from build123d import *

# Parameters (mm, degrees)
SKETCH2_R           = 22.5
SKETCH2_R_2         = 1.25
BOSS_EXTRUDE1_DEPTH = 10
SKETCH3_R           = 10
CUT_EXTRUDE1_DEPTH  = 4
FILLET1_R           = 2


with BuildPart() as part:
    # Sketch2 → Boss-Extrude1 (new body)
    with BuildSketch(Plane.XY):
        Circle(SKETCH2_R)
        with Locations((4, 0)):
            Circle(SKETCH2_R_2, mode=Mode.SUBTRACT)
        with Locations((0, 4)):
            Circle(SKETCH2_R_2, mode=Mode.SUBTRACT)
        with Locations((-4, 0)):
            Circle(SKETCH2_R_2, mode=Mode.SUBTRACT)
        with Locations((0, -4)):
            Circle(SKETCH2_R_2, mode=Mode.SUBTRACT)
    extrude(amount=BOSS_EXTRUDE1_DEPTH)

    # Sketch3 → Cut-Extrude1 (cut)
    with BuildSketch(Plane(origin=(0, 0, 0), x_dir=(-1, 0, 0), z_dir=(0, 0, -1))):
        Circle(SKETCH3_R)
    extrude(amount=-CUT_EXTRUDE1_DEPTH, mode=Mode.SUBTRACT)

    # Fillet1
    fillet1_edges = [part.edges().sort_by_distance(p)[0] for p in [
        (-22.5, 0, 0),
        (-22.5, 0, 10),
    ]]
    fillet(fillet1_edges, radius=FILLET1_R)


solid = part.part
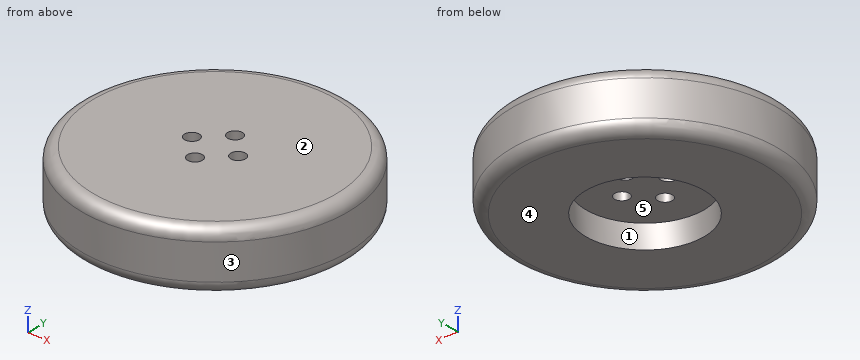
Build history of the part. All positions in model axes, mm. Face numbers are marked on the shaded views. A direction names the side the tool comes from. Round coordinates to 2 decimals unless told otherwise and drop trailing zeros. Write each loop counter-clockwise with the first axis right and the second up, starting at its lowest first coordinate (ties: lowest second). Pieces come first, ordered by that corner, then holes. Notation, with made-up numbers: M 40.5,0.5 L 90.5,0.5 A8 ccw 90.5,4.5 Z; hole C 21,-6.75 d8. An arc over 180 degrees is marked long. Answer as a JSON object with one key per item and string values. Group by question number.
(1) Which spindle directions (+Z, -Z, +X, -X, +Y, -Y) get a long thin tool onto all of the face, cutting with end or side? Do the marked faces 1 and 2. Say none if no direction does.
(2) Flat gauge pins, fed straight in: pin 1 (5 mm diameter, centred on x = 5.5, z = 2.5, fed in from -Y); pin 2 (1.5 mm diameter, centred on x = 0, y = 4, fed in from +Z); pin 3 (4 mm diameter, centred on x = -4, y = 0, fed in from -Z); pin 4 (6 mm diameter, centred on x = -16.5, z = 2, fed in from -Y). Where does each tip first touch, or does it go through?
(3) Mould opens along X. For the marked faces 3, 4 and 5 say: pulls with the +X half, pulls with the -X half, needs draft (parallel to the pull), parting line crosses it, or undercut.
(4) Cut at A-A (x = 0). Give the cut face in (y, z), and give its area (3 significant figures).
(5) Cut at C-C (z = 6.5). Give the cut face in (x, y).
(6) Drill centre lines: L1, parallel to Y at x = 0, z = 1.95; L2, parallel to Y at x = 0.5, z = 6; L3, parallel to Z at x = 9, y = -2. Where is each one in solid material? Low to high.
Responses:
{
 "1": {"face 1": "-Z", "face 2": "+Z, +X, -X, +Y, -Y"},
 "2": {"pin 1": "stops at y = -22.3", "pin 2": "passes through", "pin 3": "stops at z = 4", "pin 4": "stops at y = -18"},
 "3": {"face 3": "parting line crosses it", "face 4": "needs draft", "face 5": "undercut"},
 "4": {"outline": "M -22.5,2 A2 ccw -20.5,0 L -10,0 L -10,4 L -5.25,4 L -5.25,10 L -20.5,10 A2 ccw -22.5,8 Z; M -2.75,4 L 2.75,4 L 2.75,10 L -2.75,10 Z; M 5.25,4 L 10,4 L 10,0 L 20.5,0 A2 ccw 22.5,2 L 22.5,8 A2 ccw 20.5,10 L 5.25,10 Z", "area": "337 mm2"},
 "5": {"outline": "C 0,0 d45; hole C -4,0 d2.5; hole C 0,-4 d2.5; hole C 0,4 d2.5; hole C 4,0 d2.5"},
 "6": {"L1": "y = -22.5 to -10, 10 to 22.5", "L2": "y = -22.49 to -5.15, -2.85 to 2.85, 5.15 to 22.49", "L3": "z = 4 to 10"}
}
